from build123d import *

# Parameters (mm, degrees)
BOSS_EXTRUDE1_DEPTH   = 5
BOSS_EXTRUDE1_2_DEPTH = 5
BOSS_EXTRUDE2_DEPTH   = 2
SKETCH3_R             = 1.033864096
BOSS_EXTRUDE3_DEPTH   = 3


with BuildPart() as part:
    # Sketch1 → Boss-Extrude1 (new body)
    with BuildSketch(Plane.XY):
        Polygon((-10.505514799, 35.409303061), (-7.209900565, 31.649126626), (-5.705829991, 32.967372319), (-8.505514799, 36.161711248), (-8.505514799, 40.409303061), (-10.505514799, 40.409303061), align=None)
    extrude(amount=-BOSS_EXTRUDE1_DEPTH)



with BuildPart() as body_2:
    # Sketch1 → Boss-Extrude1 2 (new body)
    with BuildSketch(Plane.XY):
        Polygon((-13.505514799, 34.280690781), (-9.466006426, 29.671758086), (-10.970077001, 28.353512393), (-15.505514799, 33.528282595), (-15.505514799, 40.409303061), (-13.505514799, 40.409303061), align=None)
    extrude(amount=-BOSS_EXTRUDE1_2_DEPTH)


with BuildPart() as part_1:
    add(part.part)

    add(body_2.part)  # Boss-Extrude2 merges body 2
    # Sketch2 → Boss-Extrude2 (add)
    with BuildSketch(Plane.XY):
        Polygon((-10.970077001, 28.353512393), (-5.705829991, 32.967372319), (-8.505514799, 36.161711248), (-8.505514799, 40.409303061), (-15.505514799, 40.409303061), (-15.505514799, 33.528282595), align=None)
    extrude(amount=BOSS_EXTRUDE2_DEPTH)

    # Sketch3 → Boss-Extrude3 (add)
    with BuildSketch(Plane.XY.offset(2)):
        with BuildLine():
            Line((-11.57598817, 29.044835084), (-15.505514799, 33.528282595))
            Line((-15.505514799, 33.528282595), (-15.505514799, 39.490034108))
            Line((-15.505514799, 39.490034108), (-20.943415916, 34.723974688))
            ThreePointArc((-20.943415916, 34.723974688), (-22.714727935, 30.816147103), (-18.80690035, 29.044835084))
            Line((-18.80690035, 29.044835084), (-11.57598817, 29.044835084))
        make_face()
        with Locations((-19.875158133, 31.884404886)):
            Circle(SKETCH3_R, mode=Mode.SUBTRACT)
    extrude(amount=-BOSS_EXTRUDE3_DEPTH)


solid = part_1.part
Verification items for the finished model (mm, model axes). A direction names the side the tool comes from. Give positions to 0.01 mm unless a question says otherwise; leave off trailing zeros. Order: outer loops, then holes, each group sorted by start corner. A loop starts at its lowest first (then second) coordinate and runs counter-clockwise, first axis right, second up. Notation, with made-up numbers: M -24.5,-22.75 L 3.5,-22.75 A20 ccw 3.5,-13.75 Z; hole C -19.75,57.25 d1. An arc over 180 degrees is marked long. Use one line per item in the form item = value. Start each with the question number.
Q1. Go/stop test with flat-tipped pins: pin 1 Ø4 at (y, z) = (38, -3.5) entering from -X; pin 2 Ø1.5 at (y, z) = (36.5, -2.5) entering from +X; pin 3 Ø2 at (x, z) = (-12, -2) entering from -Y. Record where each tip stops, or that it passes through.
Q2. Scan lines: line 1 along X through (y, z) = (37.5, -2.5); line 2 along Y through (x, z) = (-10.25, -0.25); line 3 along X through (y, z) = (35.25, -3). Record each from-to range of solid material in increasing order. Write a range as [from, to].
Q3. Section check C-C (y = 37.5). Enter the section's corners in (x, z).
Q4. Section check B-B (z = 0.5). Enter the section's corners in (x, y).
Q5. Access from +Z, -Z, +X, -X, +Y, -Y to the whole of each face (thin tool, end or side, straight path). Record for faces 5 (the flat face through (-11.514, 32.008, -2.465)), 6 (the flat face through (-10.506, 38, -2)), 7 (the flat face through (-8.506, 38, -2)).
Q6. Mould release check, pull along X, two halves, no side actions. Record for faces 1 (the flat face through (-10, 40.409, -2)), 2 (the flat face through (-15.506, 37, -3)), 3 (the flat face through (-15, 29.045, 1)), 4 (the flat face through (-8.881, 33.556, -2.465)): +X half, -X half, draft (parallel to the pull), parting line (faces both ways), or undercut.
Q7. Section check A-A (z = -4). Enter the section's corners in (x, y).
Q8. Section check D-D (x = -10.75). Enter the section's corners in (y, z), then the cut area to 3 significant figures.
Evaluation:
q1.pin_1 = -15.51
q1.pin_2 = -8.14
q1.pin_3 = 28.39
q2.line_1 = [-15.51, -13.51], [-10.51, -8.51]
q2.line_2 = [28.98, 30.57], [35.12, 40.41]
q2.line_3 = [-15.51, -13.51], [-10.37, -7.71]
q3.outline = M -17.78,-1 L -15.51,-1 L -15.51,-5 L -13.51,-5 L -13.51,0 L -10.51,0 L -10.51,-5 L -8.51,-5 L -8.51,2 L -17.78,2 Z
q4.outline = M -20.94,34.72 A3.03 ccw -18.81,29.04 L -11.58,29.04 L -10.97,28.35 L -5.71,32.97 L -8.51,36.16 L -8.51,40.41 L -15.51,40.41 L -15.51,39.49 Z; hole C -19.88,31.88 d2.07
q5.face_5 = -Z
q5.face_6 = -Z, +Y
q5.face_7 = +Z, -Z, +X, +Y
q6.face_1 = draft
q6.face_2 = -X half
q6.face_3 = undercut
q6.face_4 = undercut
q7.outline = M -15.51,33.53 L -10.97,28.35 L -9.47,29.67 L -13.51,34.28 L -13.51,40.41 L -15.51,40.41 Z; M -10.51,35.41 L -7.21,31.65 L -5.71,32.97 L -8.51,36.16 L -8.51,40.41 L -10.51,40.41 Z
q8.outline = M 28.55,-5 L 31.14,-5 L 31.14,0 L 40.41,0 L 40.41,2 L 28.55,2 Z
q8.area = 36.7 mm2
